Verification items for this drawing (mm, ordinates from the low corner). Coordinates: 2 decimals unless noted, no trailing zeros. Loops run counter-clockwise (first coordinate to the right, second up) from the corner with the lowest first, then second, coordinate; pieces in that order, holes last. Notation, with made-up numbers: M 23.25,39.25 L 44.25,39.25 A27 cw 44.25,65.25 Z; hole C 9,28 d2. An arc over 180 degrees is marked long. Write each question's results on one line, items separated by ' | '. Start each with the question number.
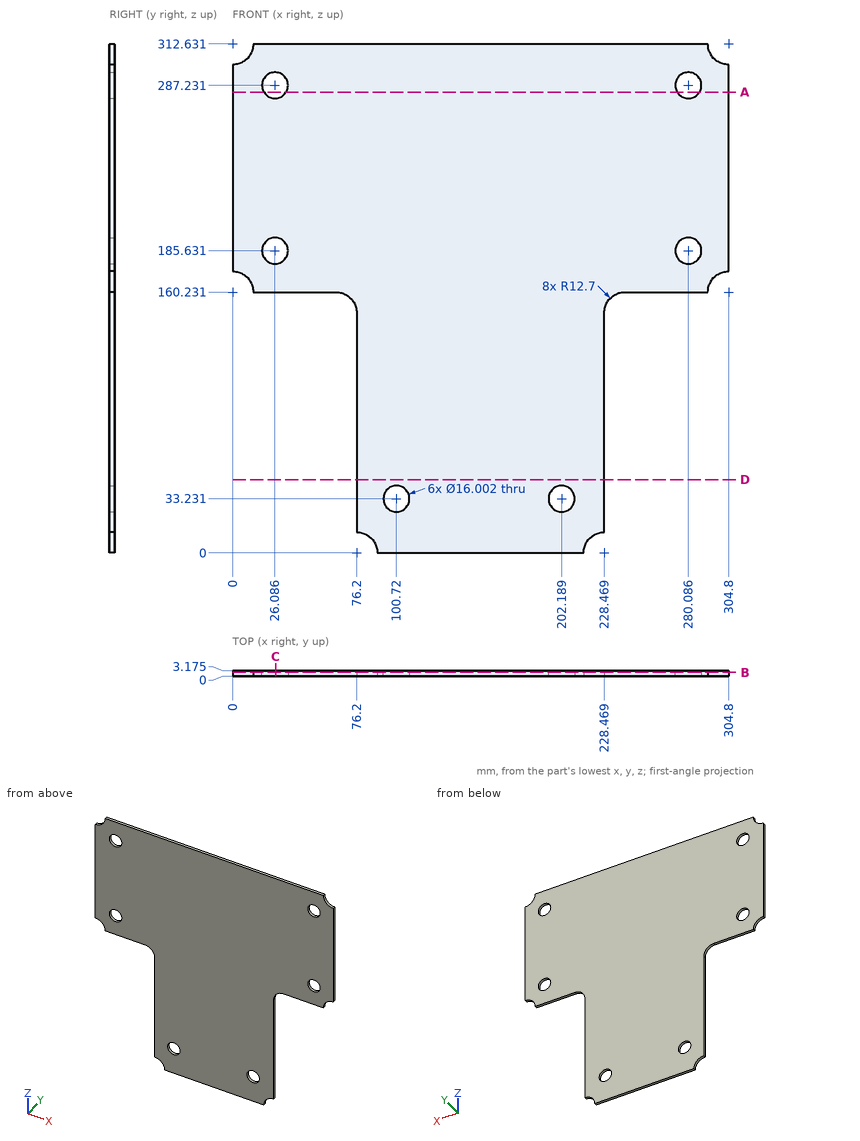
Item 1: Section check A-A (z = 283). Record the cut outline in (x, y) (1 decimal).
Item 2: Depth check by flat-ended pin: P1, Ø1.5, axis at x = 56.5, y = 2.5, coming from the -Z side; P2, Ø9.5, axis at x = 26.09, z = 287.23, coming from the -Y side. Enter the tip coordinate at first touch or a pass-through.
Item 3: Section check D-D (z = 45). Record the cut outline in (x, y) (1 decimal).
Item 4: Section check B-B (y = 2.2). Record the cut outline in (x, z) (1 decimal), plus the area to 3 significant figures.
Item 5: Section check C-C (x = 26.5). Record the cut outline in (y, z) (1 decimal).
Item 6: Thickness scan on line 1 (Z direction, x = 280, y = 1.2); line 2 (X direction, y = 2.55, z = 282); line 3 (X direction, y = 2.55, z = 137). Record the ranges inside material, lowest first.
Computed values:
1) outline: M 0,0 L 19.3,0 L 19.3,3.2 L 0,3.2 Z; M 32.9,0 L 273.3,0 L 273.3,3.2 L 32.9,3.2 Z; M 286.9,0 L 304.8,0 L 304.8,3.2 L 286.9,3.2 Z
2) P1: stops at z = 160.23 | P2: passes through
3) outline: M 76.2,0 L 228.5,0 L 228.5,3.2 L 76.2,3.2 Z
4) outline: M 0,172.9 A12.7 cw 12.7,160.2 L 63.5,160.2 A12.7 cw 76.2,147.5 L 76.2,12.7 A12.7 cw 88.9,0 L 215.8,0 A12.7 cw 228.5,12.7 L 228.5,147.5 A12.7 cw 241.2,160.2 L 292.1,160.2 A12.7 cw 304.8,172.9 L 304.8,299.9 A12.7 cw 292.1,312.6 L 12.7,312.6 A12.7 cw 0,299.9 Z; hole C 26.1,185.6 d16; hole C 26.1,287.2 d16; hole C 100.7,33.2 d16; hole C 202.2,33.2 d16; hole C 280.1,185.6 d16; hole C 280.1,287.2 d16 | area: 69,000 mm²
5) outline: M 0,160.2 L 3.2,160.2 L 3.2,177.6 L 0,177.6 Z; M 0,193.6 L 3.2,193.6 L 3.2,279.2 L 0,279.2 Z; M 0,295.2 L 3.2,295.2 L 3.2,312.6 L 0,312.6 Z
6) line 1: z = 160.23 to 177.63, 193.63 to 279.23, 295.23 to 312.63 | line 2: x = 0 to 20.03, 32.14 to 274.03, 286.14 to 304.8 | line 3: x = 76.2 to 228.47
